Design review of the part built by this model. Coordinates are the model's own, in mm. Give positions to 0.01 mm unless a question says otherwise; leave off trailing zeros. Write each loop counter-clockwise with the first axis right and the second up, starting at its lowest first coordinate (ties: lowest second). Pieces come first, ordered by that corner, then holes.
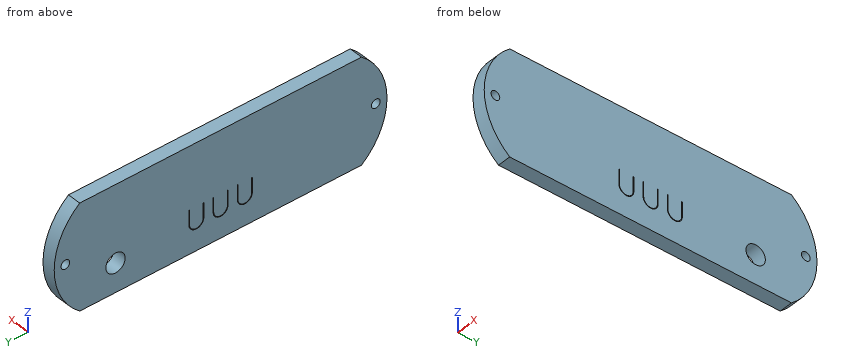
```python
from build123d import *

# Parameters (mm, degrees)
F0_R     = 4.05
F0_R_2   = 1.8288
F1_DEPTH = 5.588
F3_DEPTH = 5.588


with BuildPart() as f1:
    # F0 (on Right) → F1 (new body)
    with BuildSketch(Plane.YZ):
        with BuildLine():
            ThreePointArc((59, -22), (69.679492, 0), (59, 22))
            Line((59, 22), (-59, 22))
            ThreePointArc((-59, 22), (-69.679492, 0), (-59, -22))
            Line((-59, -22), (59, -22))
        make_face()
        with Locations((44, -9.95)):
            Circle(F0_R, mode=Mode.SUBTRACT)
        with Locations((-65, 0)):
            Circle(F0_R_2, mode=Mode.SUBTRACT)
        with Locations((65, 0)):
            Circle(F0_R_2, mode=Mode.SUBTRACT)
    extrude(amount=F1_DEPTH)

    # F2 (on face) → F3 (cut, through all)
    with BuildSketch(Plane.YZ.offset(5.588)):
        with BuildLine():
            ThreePointArc((7.287, -4), (7.16, -3.873), (7.033, -4))
            Line((7.033, -4), (7.033, -10))
            ThreePointArc((7.033, -10), (10.16, -13.127), (13.287, -10))
            Line((13.287, -10), (13.287, -4))
            ThreePointArc((13.287, -4), (13.16, -3.873), (13.033, -4))
            Line((13.033, -4), (13.033, -10))
            ThreePointArc((13.033, -10), (10.16, -12.873), (7.287, -10))
            Line((7.287, -10), (7.287, -4))
        make_face()
        with BuildLine():
            ThreePointArc((2.873, -10), (0, -12.873), (-2.873, -10))
            Line((-2.873, -10), (-2.873, -4))
            ThreePointArc((-2.873, -4), (-3, -3.873), (-3.127, -4))
            Line((-3.127, -4), (-3.127, -10))
            ThreePointArc((-3.127, -10), (0, -13.127), (3.127, -10))
            Line((3.127, -10), (3.127, -4))
            ThreePointArc((3.127, -4), (3, -3.873), (2.873, -4))
            Line((2.873, -4), (2.873, -10))
        make_face()
        with BuildLine():
            ThreePointArc((-7.287, -10), (-10.16, -12.873), (-13.033, -10))
            Line((-13.033, -10), (-13.033, -4))
            ThreePointArc((-13.033, -4), (-13.16, -3.873), (-13.287, -4))
            Line((-13.287, -4), (-13.287, -10))
            ThreePointArc((-13.287, -10), (-10.16, -13.127), (-7.033, -10))
            Line((-7.033, -10), (-7.033, -4))
            ThreePointArc((-7.033, -4), (-7.16, -3.873), (-7.287, -4))
            Line((-7.287, -4), (-7.287, -10))
        make_face()
    extrude(amount=-F3_DEPTH, mode=Mode.SUBTRACT)


solid = f1.part
```
(1) To check wall thickness, follow L1, parallel to Y at x = 2.9, z = 1.5; L2, parallel to Z at x = 4.45, y = 63.5; L3, parallel to Z at x = 3.4, y = 65. State the ranges of each line that lie inside material, in increasing order.
Resolved:
L1: y = -69.64 to -66.05, -63.95 to 63.95, 66.05 to 69.64
L2: z = -17.55 to -1.05, 1.05 to 17.55
L3: z = -15.5 to -1.83, 1.83 to 15.5
(2) Consider section B-B, the plane y = 44. Give the boundary of the cut face in (x, z), then the cut area to 3 significant figures.
Resolved:
outline: (0, -22) - (5.59, -22) - (5.59, -14) - (0, -14) - close; (0, -5.9) - (5.59, -5.9) - (5.59, 22) - (0, 22) - close
area: 201 mm2
(3) Clearance check with flat-ended pins moving along their axes: P1, Ø3, axis at y = 65, z = 0, coming from the +X side; P2, Ø3, axis at x = 2.5, z = -8, coming from the +Y side; P3, Ø2, axis at x = 2, z = 8.5, coming from the -Y side; P4, Ø3, axis at x = 3, z = -7, coming from the -Y side. State where each tip first meets the part, or that it passes through.
Resolved:
P1: passes through
P2: stops at y = 68.91
P3: stops at y = -68.66
P4: stops at y = -69.13
(4) Consider section C-C, the plane y = 65. Give the boundary of the cut face in (x, z).
Resolved:
outline: (0, -15.5) - (5.59, -15.5) - (5.59, -1.83) - (0, -1.83) - close; (0, 1.83) - (5.59, 1.83) - (5.59, 15.5) - (0, 15.5) - close
(5) Consider section A-A, the plane x = 0.9. Give the number of separate pieces and of enclosed holes in the cut face, then the cut area to 3 significant figures.
Resolved:
separate pieces: 1
enclosed holes: 6
area: 5,760 mm2
